Geometry check sheet. Reference: the model listing, model coordinates, mm. Face numbers are marked on the shaded views. A direction names the side the tool comes from. Coordinates: 2 decimals unless noted, no trailing zeros. Loops run counter-clockwise (first coordinate to the right, second up) from the corner with the lowest first, then second, coordinate; pieces in that order, holes last. Notation, with made-up numbers: (29.5, 61.5) - (87.5, 61.5) arc R25 cw to (87.5, 99.5) - close; hole circle Ø3 at (-34.5, 54.25). An arc over 180 degrees is marked (long way). One line per item, written item: value.
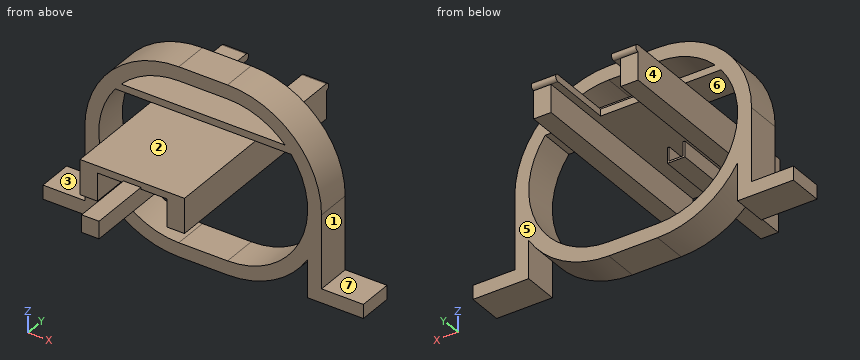
from build123d import *

# Parameters (mm, degrees)
EXTRUDE_1_DEPTH     = 10
SKETCH_3_W          = 30
SKETCH_3_H          = 60
EXTRUDE_2_DEPTH     = 10
SKETCH_7_R          = 1
EXTRUDE_4_DEPTH     = 30
SKETCH_6_W          = 16
SKETCH_6_H          = 49.282767792
CUT_EXTRUDE_2_DEPTH = 24
SKETCH_8_W          = 20
SKETCH_8_H          = 68.65426033
CUT_EXTRUDE_3_DEPTH = 8
SKETCH_10_W         = 4
SKETCH_10_H         = 4
SKETCH_16_W         = 5
SKETCH_16_H         = 5
EXTRUDE_5_DEPTH     = 2
SKETCH_17_W         = 4
SKETCH_17_H         = 25
EXTRUDE_6_DEPTH     = 10
SKETCH_18_W         = 12
SKETCH_18_H         = 4
EXTRUDE_7_DEPTH     = 10


with BuildPart() as part:
    # 草图2 → 凸台-拉伸1 (new body)
    with BuildSketch(Plane(origin=(0, 0, 0), x_dir=(1, 0, 0), z_dir=(0, 1, 0))):
        with BuildLine():
            Line((-7, 27), (7, 27))
            ThreePointArc((7, 27), (34, 0), (7, -27))
            Line((7, -27), (-7, -27))
            ThreePointArc((-7, -27), (-34, 0), (-7, 27))
        make_face()
        with BuildLine():
            Line((-7, 23), (7, 23))
            ThreePointArc((7, 23), (27.627651345, 10.173494975), (25.248287591, -14))
            Line((25.248287591, -14), (-25.248287591, -14))
            ThreePointArc((-25.248287591, -14), (-27.627651345, 10.173494975), (-7, 23))
        make_face(mode=Mode.SUBTRACT)
        with BuildLine():
            Line((-7, -23), (7, -23))
            ThreePointArc((7, -23), (15.972179222, -21.177818585), (23.522711642, -16))
            Line((23.522711642, -16), (-23.522711642, -16))
            ThreePointArc((-23.522711642, -16), (-15.972179222, -21.177818585), (-7, -23))
        make_face(mode=Mode.SUBTRACT)
    extrude(amount=EXTRUDE_1_DEPTH)

    # 草图3 → 凸台-拉伸2 (add)
    with BuildSketch(Plane(origin=(0, 0, 14), x_dir=(-1, 0, 0), z_dir=(0, 0, -1))):
        Rectangle(SKETCH_3_W, SKETCH_3_H)
    extrude(amount=EXTRUDE_2_DEPTH)

    # 草图7 → 凸台-拉伸4 (add)
    with BuildSketch(Plane.ZY.offset(15)):
        with Locations((13, 30)):
            Circle(SKETCH_7_R)
    extrude(amount=-EXTRUDE_4_DEPTH)

    # 草图6 → 切除-拉伸2 (cut, through all)
    with BuildSketch(Plane(origin=(0, 0, 4), x_dir=(-1, 0, 0), z_dir=(0, 0, -1))):
        with Locations((0, 36.641383896)):
            Rectangle(SKETCH_6_W, SKETCH_6_H)
    extrude(amount=-CUT_EXTRUDE_2_DEPTH, mode=Mode.SUBTRACT)

    # 草图8 → 切除-拉伸3 (cut)
    with BuildSketch(Plane(origin=(0, 0, 4), x_dir=(-1, 0, 0), z_dir=(0, 0, -1))):
        with Locations((0, -1.849037214)):
            Rectangle(SKETCH_8_W, SKETCH_8_H)
    extrude(amount=-CUT_EXTRUDE_3_DEPTH, mode=Mode.SUBTRACT)

    # 扫描2: sweep along a path in 草图12
    with BuildLine(Plane(origin=(0, 0, 12), x_dir=(-1, 0, 0), z_dir=(0, 0, -1))) as sweep_2_path:
        Line((-2.5, -8.196811454), (-2.5, -45.72167139))
    # 草图10 → 扫描2 (sweep)
    with BuildSketch(Plane.XZ.offset(30)):
        Polygon((-2.5, 12), (-2.5, 7.5), (2.5, 7.5), (2.5, 12), (2.5, 12.5), (-2.5, 12.5), align=None)
        with Locations((0, 10)):
            Rectangle(SKETCH_10_W, SKETCH_10_H, mode=Mode.SUBTRACT)
    sweep(path=sweep_2_path.line)

    # 草图16 → 凸台-拉伸5 (add)
    with BuildSketch(Plane.XZ.offset(45.72167139)):
        with Locations((0, 10)):
            Rectangle(SKETCH_16_W, SKETCH_16_H)
    extrude(amount=EXTRUDE_5_DEPTH)

    # 草图17 → 凸台-拉伸6 (add)
    with BuildSketch(Plane(origin=(0, 10, 0), x_dir=(1, 0, 0), z_dir=(0, 1, 0))):
        with Locations((-32, 12.5)):
            Rectangle(SKETCH_17_W, SKETCH_17_H)
        with Locations((32, 12.5)):
            Rectangle(SKETCH_17_W, SKETCH_17_H)
    extrude(amount=-EXTRUDE_6_DEPTH)

    # 草图18 → 凸台-拉伸7 (add)
    with BuildSketch(Plane(origin=(0, 10, 0), x_dir=(1, 0, 0), z_dir=(0, 1, 0))):
        with Locations((-40, 23)):
            Rectangle(SKETCH_18_W, SKETCH_18_H)
        with Locations((40, 23)):
            Rectangle(SKETCH_18_W, SKETCH_18_H)
    extrude(amount=-EXTRUDE_7_DEPTH)


solid = part.part
(1) Cross-section at A-A on y = -13.5. Record the cut outline in (x, z).
Reply:
outline: (-15, 4) - (-10, 4) - (-10, 12) - (-2.5, 12) - (-2.5, 7.5) - (2.5, 7.5) - (2.5, 12) - (10, 12) - (10, 4) - (15, 4) - (15, 14) - (-15, 14) - close; hole (-2, 8) - (2, 8) - (2, 12) - (-2, 12) - close
(2) Material ranges on probe 1 along X at (y, z) = (-18.5, 11); probe 2 along X at (y, z) = (12, 6.5); probe 3 along Z at (x, y) = (4, 2.5), recorded low to high. Write a range as from..to.
Reply:
probe 1: -15..-10, -2.5..-2, 2..2.5, 10..15
probe 2: -15..-10, 10..15
probe 3: -27..-23, 12..16, 23..27
(3) Cross-section at C-C on y = 18.5. Record the cut outline in (x, z).
Reply:
outline: (-15, 4) - (-10, 4) - (-10, 12) - (-8, 12) - (-8, 14) - (-15, 14) - close; (8, 12) - (10, 12) - (10, 4) - (15, 4) - (15, 14) - (8, 14) - close
(4) Cross-section at B-B on x = 13.5. Record the cut outline in (y, z).
Reply:
outline: (-30, 4) - (30, 4) - (30, 12) arc R1 ccw to (30, 14) - (10, 14) - (10, 16) - (0, 16) - (0, 14) - (-30, 14) - close; (0, -26.21) - (10, -26.21) - (10, -22.06) - (0, -22.06) - close; (0, 22.06) - (10, 22.06) - (10, 26.21) - (0, 26.21) - close
(5) Go/stop test with flat-tipped pins: pin 1 Ø2 at (x, z) = (14, 5) entering from -Y; pin 2 Ø4.5 at (y, z) = (-31, 10.5) entering from -X; pin 3 Ø5.5 at (y, z) = (-27.5, 10) entering from +X. Record where each tip stops, or that it passes through.
Reply:
pin 1: y = -30
pin 2: x = -15
pin 3: x = 15
(6) Access from +Z, -Z, +X, -X, +Y, -Y to the whole of each face (thin tool, end or side, straight path). Record for the marked faces 1, 2, 3 and 4.
Reply:
face 1: +Z, +X, +Y, -Y
face 2: +Z, +X, -X, -Y
face 3: +Z, -X, +Y, -Y
face 4: +Y, -Y
(7) Release check for a two-part mould opening along Z. For the marked faces 5, 6 and 7 record: pulls with the +Z half, pulls with the -Z half, needs draft (parallel to the pull), parting line crosses it, or undercut.
Reply:
face 5: needs draft
face 6: undercut
face 7: pulls with the +Z half
(8) Cross-section at D-D on z = 21. Record the cut outline in (x, y).
Reply:
outline: (-23.97, 0) - (-16.38, 0) - (-16.38, 10) - (-23.97, 10) - close; (16.38, 0) - (23.97, 0) - (23.97, 10) - (16.38, 10) - close
